Input: part model. Units: mm. Frame: model coordinates. Give positions to 0.01 mm unless a question says otherwise; leave off trailing zeros. Order: outer loops, then holes, each group sorted by start corner. A loop starts at its lowest first (then second) coordinate and runs counter-clockwise, first axis right, second up. Notation, with made-up numbers: (-21.75, -9) - (19.25, -9) arc R26 ccw to (19.25, 25) - close; hole circle Ø3 at (-26.5, -31.5). An arc over 180 degrees is marked (long way). Answer in a Markdown table with one row per item. Add a question column.
1. Section query A-A on x = 7.5. Return loops of the section in (y, z).
2. Contact query for a flat-ended pin moving along its axis: pin 1 (4 mm diameter, centred on x = -10.75, y = -35.75, fed in from +Z). Output: stop coordinate, or through.
3. Ray query, line 1 (X direction, y = 14, z = 1.9); line 2 (Y direction, x = -11, z = 0.6); line 3 (Y direction, x = 8, z = 2.45). Return the intervals inside material, ascending. Write a range as [from, to].
4. Section query B-B on z = 0.6. Count the separate pieces of the cut face and the enclosed holes in it, and give its area (3 significant figures).
Autodesk Fusion 360 part; units mm, degrees
sketch "Esquisse1" plane through (0, 0, 0) normal (0, 0, 1) x (1, 0, 0)
  line L0 (75, -53) -> (-75, -53)
  line L1 (-75, -53) -> (-75, 53)
  line L2 (-75, 53) -> (75, 53)
  line L3 (75, 53) -> (75, -53)
  line L4 (75, -53) -> (-75, 53) construction
  line L5 (-75, -53) -> (75, 53) construction
  line L6 (78, 50) -> (-78, 50)
  line L7 (-78, 50) -> (-78, -50)
  line L8 (-78, -50) -> (78, -50)
  line L9 (78, -50) -> (78, 50)
  line L10 (78, 50) -> (-78, -50) construction
  line L11 (-78, 50) -> (78, -50) construction
  dimension "d1" = 150
  dimension "d2" = 106
  dimension "d49" = 156
  dimension "d50" = 100
extrude "Extrusion1" add sketch "Esquisse1" along normal blind 3
sketch "Esquisse4" plane through (0, 0, 3) normal (0, 0, 1) x (-1, 0, 0)
  line L0 (-75, -53) -> (75, -53)
  line L1 (75, -53) -> (75, -50)
  line L2 (75, 53) -> (-75, 53)
  line L3 (-75, -50) -> (-75, -53)
  circle A0 centre (-25, -37.5) radius 2.5
  circle A1 centre (-25, -28.125) radius 2.5
  circle A2 centre (-25, -18.75) radius 2.5
  circle A3 centre (-25, -9.375) radius 2.5
  circle A4 centre (-25, 0) radius 2.5
  circle A5 centre (-12.1742, -35.2385) radius 2.5
  circle A6 centre (-0.8955, -28.7267) radius 2.5
  circle A7 centre (7.476, -18.75) radius 2.5
  circle A8 centre (11.9303, -6.5118) radius 2.5
  circle A9 centre (11.9303, 6.5118) radius 2.5
  circle A10 centre (7.476, 18.75) radius 2.5
  circle A11 centre (-0.8955, 28.7267) radius 2.5
  circle A12 centre (-12.1742, 35.2385) radius 2.5
  circle A13 centre (-25, 37.5) radius 2.5
  circle A14 centre (-37.8258, 35.2385) radius 2.5
  circle A15 centre (-49.1045, 28.7267) radius 2.5
  circle A16 centre (-57.476, 18.75) radius 2.5
  circle A17 centre (-61.9303, 6.5118) radius 2.5
  circle A18 centre (-61.9303, -6.5118) radius 2.5
  circle A19 centre (-57.476, -18.75) radius 2.5
  circle A20 centre (-49.1045, -28.7267) radius 2.5
  circle A21 centre (-37.8258, -35.2385) radius 2.5
  circle A22 centre (-12.797, -25.3397) radius 2.5
  circle A23 centre (-3.011, -17.5357) radius 2.5
  circle A24 centre (2.4198, -6.2584) radius 2.5
  circle A25 centre (2.4198, 6.2584) radius 2.5
  circle A26 centre (-3.011, 17.5357) radius 2.5
  circle A27 centre (-12.797, 25.3397) radius 2.5
  circle A28 centre (-25, 28.125) radius 2.5
  circle A29 centre (-37.203, 25.3397) radius 2.5
  circle A30 centre (-46.989, 17.5357) radius 2.5
  circle A31 centre (-52.4198, 6.2584) radius 2.5
  circle A32 centre (-52.4198, -6.2584) radius 2.5
  circle A33 centre (-46.989, -17.5357) radius 2.5
  circle A34 centre (-37.203, -25.3397) radius 2.5
  circle A35 centre (-13.979, -15.1691) radius 2.5
  circle A36 centre (-7.1677, -5.7941) radius 2.5
  circle A37 centre (-7.1677, 5.7941) radius 2.5
  circle A38 centre (-13.979, 15.1691) radius 2.5
  circle A39 centre (-25, 18.75) radius 2.5
  circle A40 centre (-36.021, 15.1691) radius 2.5
  circle A41 centre (-42.8323, 5.7941) radius 2.5
  circle A42 centre (-42.8323, -5.7941) radius 2.5
  circle A43 centre (-36.021, -15.1691) radius 2.5
  circle A44 centre (-17.6703, -5.8452) radius 2.5
  circle A45 centre (-15.8601, 2.0861) radius 2.5
  circle A46 centre (-20.9323, 8.4466) radius 2.5
  circle A47 centre (-29.0677, 8.4466) radius 2.5
  circle A48 centre (-34.1399, 2.0861) radius 2.5
  circle A49 centre (-32.3297, -5.8452) radius 2.5
  line L4 (-75, 50) -> (-78, 50)
  line L5 (-78, 50) -> (-78, -50)
  line L6 (-78, -50) -> (-75, -50)
  line L7 (75, -50) -> (78, -50)
  line L8 (78, -50) -> (78, 50)
  line L9 (78, 50) -> (75, 50)
  line L10 (75, 50) -> (75, 53)
  line L11 (-75, 53) -> (-75, 50)
  circle A50 centre (-60.75, -35.75) radius 2.2
  circle A51 centre (10.75, 35.75) radius 2.2
  line L12 (-60.75, -35.75) -> (10.75, -35.75)
  line L13 (10.75, 35.75) -> (-60.75, -35.75) construction
  line L14 (-60.75, 35.75) -> (10.75, -35.75) construction
  circle A52 centre (10.75, -35.75) radius 2.2
  line L15 (10.75, 35.75) -> (-60.75, 35.75)
  line L16 (-60.75, 35.75) -> (-60.75, -35.75)
  line L17 (10.75, -35.75) -> (10.75, 35.75)
  circle A53 centre (-60.75, 35.75) radius 2.2
  line L18 (-75, 50) -> (-78, 50)
  point P0 (-25, 0)
  dimension "d32" = 5
  dimension "d37" = 0
  dimension "d38" = 37.5
  dimension "d40" = 360
  dimension "d42" = 360
  dimension "d44" = 360
  dimension "d46" = 360
  dimension "d51" = 71.5
  dimension "d52" = 71.5
  dimension "d53" = 4.4
  dimension "d54" = 4.4
  dimension "d55" = 4.4
  dimension "d56" = 4.4
extrude "Extrusion5" cut sketch "Esquisse4" against normal blind 3 contours A0 L12 | A0 L12 | A5 L12 | A5 L12 | A21 L12 | A21 L12 | L12 A52 L17 | L12 A52 L17 | A50 L12 L16 | A50 L12 L16 | A8 L17 | A8 L17 | A18 L16 | A18 L16 | A9 L17 | A9 L17 | A17 L16 | A17 L16 | A51 L15 L17 | A51 L15 L17 | L15 L16 A53 | L15 L16 A53 | A12 L15 | A12 L15 | A14 L15 | A14 L15 | A13 L15 | A13 L15 | A1 | A2 | A3 | A4 | A6 | A7 | A10 | A11 | A15 | A16 | A19 | A20 | A22 | A23 | A24 | A25 | A26 | A27 | A28 | A29 | A30 | A31 | A32 | A33 | A34 | A35 | A36 | A37 | A38 | A39 | A40 | A41 | A42 | A43 | A44 | A45 | A46 | A47 | A48 | A49
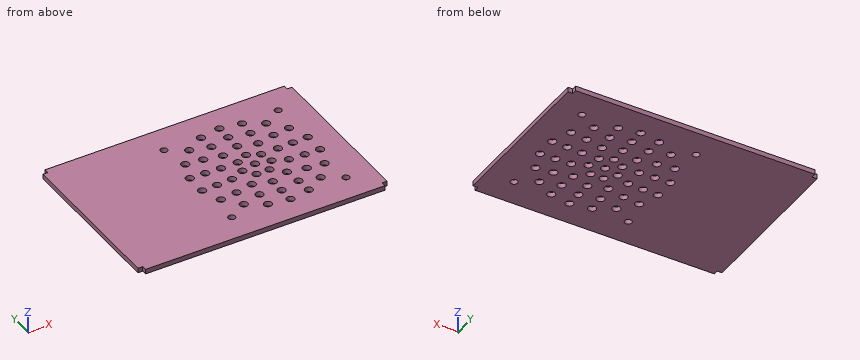
Answer:
| question | item | result |
|---|---|---|
| 1 | outline | (-53, 0) - (-8.27, 0) - (-8.27, 3) - (-53, 3) - close; (-3.32, 0) - (3.32, 0) - (3.32, 3) - (-3.32, 3) - close; (8.27, 0) - (53, 0) - (53, 3) - (8.27, 3) - close |
| 2 | pin 1 | passes through |
| 3 | line 1 | x = [-78, 11.77], [16.19, 33.81], [38.23, 78] |
| 3 | line 2 | y = [-53, -37.94], [-33.56, -8.83], [-4.19, 4.19], [8.83, 33.56], [37.94, 53] |
| 3 | line 3 | y = [-53, -8.15], [-3.44, 3.44], [8.15, 53] |
| 4 | separate pieces | 1 |
| 4 | enclosed holes | 54 |
| 4 | area | 15,500 mm² |
